CAD build for the part. Positions are in the model's coordinates, mm. A direction names the side the tool comes from. Round coordinates to 2 decimals unless told otherwise and drop trailing zeros. Write each loop counter-clockwise with the first axis right and the second up, starting at its lowest first coordinate (ties: lowest second). Pieces come first, ordered by that corner, then holes. Notation, with made-up numbers: (19, 63) -> (71, 63) arc R31 cw to (71, 92) -> close; hole circle Ø7 at (34, 78). An arc over 180 degrees is marked (long way). Put each result on its own line as item: value. Start each with the question number.
1. 3-axis set-ups, long thin cutter, end or side, ignore diameter. For faces 1 (the flat face through (-7, -1, -1)), 2 (the cylindrical face through (-15.65, -0.06, -1.23)), 3 (the cylindrical face through (-6.604, 2.421, 1.183)), 4 (the cylindrical face through (15.65, 0.06, -1.23)), 5 (the cylindrical face through (-0.73, -3.32, -1.23)): which of +Z, -Z, +X, -X, +Y, -Y reach the whole face in a straight line?
2. Pull direction Y, two halves, no side cores. Call faces 6 (the cylindrical face through (6.604, -2.421, 1.183)), 7 (the cylindrical face through (-3.918, 4.953, -0.873)), 8 (the flat face through (0, 0, -2.5)): pulls with the +Y half, pulls with the -Y half, needs draft (parallel to the pull), parting line crosses it, or undercut.
3. Saw through at B-B on y = -9.5. List the corners of the cut face in (x, z), and give its area (3 significant figures).
4. Drill centre lines: line 1 (Y direction, x = -9.5, z = -0.25); line 2 (X direction, y = 4.5, z = -1.4); line 3 (Z direction, x = 1.5, y = 15.5). Where is each one in solid material? Low to high. Write a range as from..to.
5. Flat gauge pins, fed straight in: P1, Ø2, axis at x = 0.5, z = -0.5, coming from the +Y side; P2, Ø1, axis at y = -6, z = -1, coming from the +X side; P3, Ø2, axis at x = 9, z = -1, coming from the -Y side. Where does each tip first touch, or does it go through?
6. Saw through at A-A on x = -9.5. List the corners of the cut face in (y, z).
7. Saw through at D-D on x = -14.5. List the corners of the cut face in (y, z), and give its area (3 significant figures).
8. Saw through at C-C on x = 0. List the corners of the cut face in (y, z).
from build123d import *

# Parameters (mm, degrees)
F1_DEPTH = 2.5
F2_R     = 2.5
F2_R_2   = 3.5
F3_DEPTH = 1
F4_DEPTH = 25
F6_DEPTH = 2.4
F7_DEPTH = 0.8
F8_ANGLE = 180


with BuildPart() as f1:
    # F0 (on Top) → F1 (new body)
    with BuildSketch(Plane.XY):
        with BuildLine():
            ThreePointArc((-17.7467741935, 3.8045375176), (-15.65, 0), (-17.7467741935, -3.8045375176))
            ThreePointArc((-17.7467741935, -3.8045375176), (0, -18.15), (17.7467741935, -3.8045375176))
            ThreePointArc((17.7467741935, -3.8045375176), (15.65, 0), (17.7467741935, 3.8045375176))
            ThreePointArc((17.7467741935, 3.8045375176), (0, 18.15), (-17.7467741935, 3.8045375176))
        make_face()
        with BuildLine():
            ThreePointArc((2.4959380946, -2.3087427375), (5.3934479575, -2.1979674519), (5.5, -5.0956356923))
            ThreePointArc((5.5, -5.0956356923), (1.7016498657, -7.3374880505), (-2.7, -7.0566959612))
            ThreePointArc((-2.7, -7.0566959612), (-3.9459149151, -4.3705658168), (-1.241297598, -3.1653088749))
            ThreePointArc((-1.241297598, -3.1653088749), (0.7595769091, -3.3140674283), (2.4959380946, -2.3087427375))
        make_face(mode=Mode.SUBTRACT)
        with BuildLine():
            ThreePointArc((-8.7553190403, 9.1305469991), (0.952140072, 12.6141162704), (10.0266934622, 7.7128411247))
            ThreePointArc((10.0266934622, 7.7128411247), (9.5115151335, 3.7722871727), (5.5712685972, 4.2898114644))
            Line((5.5712685972, 4.2898114644), (5.5118136083, 4.3702173366))
            ThreePointArc((5.5118136083, 4.3702173366), (3.8930445069, 4.946510168), (2.7952312611, 3.6246429626))
            ThreePointArc((2.7952312611, 3.6246429626), (2.3794320778, 2.9889401783), (1.6198224227, 2.9893436268))
            ThreePointArc((1.6198224227, 2.9893436268), (-0.1325337371, 3.3974159016), (-1.8477750037, 2.8540720972))
            ThreePointArc((-1.8477750037, 2.8540720972), (-4.009187674, 2.5898113989), (-5.5508583046, 4.1275988078))
            ThreePointArc((-5.5508583046, 4.1275988078), (-5.9755788699, 4.654107591), (-6.6382950389, 4.7897775457))
            ThreePointArc((-6.6382950389, 4.7897775457), (-9.2794977325, 6.1882728138), (-8.7553190403, 9.1305469991))
        make_face(mode=Mode.SUBTRACT)
    extrude(amount=F1_DEPTH)

    # F2 (on face) → F3 (cut)
    with BuildSketch(Plane(origin=(0, 0, 0), x_dir=(1, 0, 0), z_dir=(0, 0, -1))):
        with BuildLine():
            ThreePointArc((9.0125481144, -3.4658895913), (11.7960747375, -2.6415981526), (13, 0))
            ThreePointArc((13, 0), (7.5843636972, 2.9292213224), (8.0969499684, -3.2064701166))
            ThreePointArc((8.0969499684, -3.2064701166), (8.5658137707, -3.297127868), (9.0125481144, -3.4658895913))
        make_face()
        with Locations((9.5, 0)):
            Circle(F2_R, mode=Mode.SUBTRACT)
        with Locations((-9.5, 0)):
            Circle(F2_R_2)
        with Locations((-9.5, 0)):
            Circle(F2_R, mode=Mode.SUBTRACT)
    extrude(amount=-F3_DEPTH, mode=Mode.SUBTRACT)

    # F2 (on face) → F4 (cut)
    with BuildSketch(Plane(origin=(0, 0, 0), x_dir=(1, 0, 0), z_dir=(0, 0, -1))):
        with Locations((9.5, 0)):
            Circle(F2_R)
        with Locations((-9.5, 0)):
            Circle(F2_R)
    extrude(amount=-F4_DEPTH, mode=Mode.SUBTRACT)

    # F5 (on face) → F6 (join)
    with BuildSketch(Plane(origin=(0, 0, 0), x_dir=(1, 0, 0), z_dir=(0, 0, -1))):
        with BuildLine():
            ThreePointArc((6.0601535804, -3.7943429711), (6.2633893685, -3.4485436953), (6.4469143417, -3.0918918919))
            ThreePointArc((6.4469143417, -3.0918918919), (6.6042114466, -2.4108440907), (6.4561602608, -1.7277267266))
            ThreePointArc((6.4561602608, -1.7277267266), (6.4124110495, -1.6482701455), (6.3707355238, -1.5677065536))
            ThreePointArc((6.3707355238, -1.5677065536), (4.9243798524, -0.8019946659), (3.5615820489, -1.7081081081))
            ThreePointArc((3.5615820489, -1.7081081081), (3.1023693948, -2.4449548335), (2.4932688314, -3.0636759839))
            ThreePointArc((2.4932688314, -3.0636759839), (2.7026586012, -3.3127187828), (2.7952312611, -3.6246429626))
            ThreePointArc((2.7952312611, -3.6246429626), (3.8930445069, -4.946510168), (5.5118136083, -4.3702173366))
            Line((5.5118136083, -4.3702173366), (5.5712685972, -4.2898114644))
            ThreePointArc((5.5712685972, -4.2898114644), (5.8003063385, -4.0268771571), (6.0601535804, -3.7943429711))
        make_face()
        with BuildLine():
            ThreePointArc((3.8959765845, -5.9953203795), (5.0982553244, -5.0130123326), (6.0601535804, -3.7943429711))
            ThreePointArc((6.0601535804, -3.7943429711), (5.8003063385, -4.0268771571), (5.5712685972, -4.2898114644))
            Line((5.5712685972, -4.2898114644), (5.5118136083, -4.3702173366))
            ThreePointArc((5.5118136083, -4.3702173366), (3.8930445069, -4.946510168), (2.7952312611, -3.6246429626))
            ThreePointArc((2.7952312611, -3.6246429626), (2.7026586012, -3.3127187828), (2.4932688314, -3.0636759839))
            ThreePointArc((2.4932688314, -3.0636759839), (2.3261145429, -3.192442816), (2.1523227285, -3.3121000698))
            ThreePointArc((2.1523227285, -3.3121000698), (1.6825395016, -5.5255371527), (3.8959765845, -5.9953203795))
        make_face()
        with BuildLine():
            ThreePointArc((-3.8662701246, 6.0141635011), (-3.8811751433, 6.0048235859), (-3.8959765845, 5.9953203795))
            ThreePointArc((-3.8959765845, 5.9953203795), (-5.3713427021, 4.7192348508), (-6.4469143417, 3.0918918919))
            ThreePointArc((-6.4469143417, 3.0918918919), (-6.6042114466, 2.4108440907), (-6.4561602608, 1.7277267266))
            ThreePointArc((-6.4561602608, 1.7277267266), (-6.4124110495, 1.6482701455), (-6.3707355238, 1.5677065536))
            ThreePointArc((-6.3707355238, 1.5677065536), (-4.9243798524, 0.8019946659), (-3.5615820489, 1.7081081081))
            ThreePointArc((-3.5615820489, 1.7081081081), (-3.0956887113, 2.4534081198), (-2.4765181166, 3.0772322009))
            ThreePointArc((-2.4765181166, 3.0772322009), (-3.8784449822, 4.2111223181), (-3.8662701246, 6.0141635011))
        make_face()
        with BuildLine():
            ThreePointArc((-2.1523227285, 3.3121000698), (-1.6730362952, 5.5107357114), (-3.8662701246, 6.0141635011))
            ThreePointArc((-3.8662701246, 6.0141635011), (-3.8784449822, 4.2111223181), (-2.4765181166, 3.0772322009))
            ThreePointArc((-2.4765181166, 3.0772322009), (-2.3173978125, 3.1987759188), (-2.1523227285, 3.3121000698))
        make_face()
    extrude(amount=F6_DEPTH)

    # F7 (cut): faces of the model
    f7_faces = [f1.faces().sort_by_distance(p)[0] for p in [
        (2.880203055, 4.9455389585, 0),
        (-2.7641546482, -4.7635377555, 0),
    ]]
    extrude(f7_faces, amount=-F7_DEPTH, mode=Mode.SUBTRACT)


with BuildPart() as f1_1:
    # F8: moved
    add(f1.part.rotate(Axis((0, 0, 0), (0, -1, 0)), F8_ANGLE))


solid = f1_1.part
Return value:
1. face 1: +Z
1. face 2: +Z, -Z, -X
1. face 3: +Z, -X
1. face 4: +Z, -Z, +X
1. face 5: +Z, -Z
2. face 6: parting line crosses it
2. face 7: undercut
2. face 8: needs draft
3. outline: (-15.47, -2.5) -> (15.47, -2.5) -> (15.47, 0) -> (-15.47, 0) -> close
3. area: 77.3 mm^2
4. line 1: y = -15.47..-3.5, 3.5..3.76, 8.35..15.47
4. line 2: x = -17.58..-10.18, -5.41..-3.17, 5.78..17.58
4. line 3: z = -2.5..0
5. P1: stops at y = 18.15
5. P2: stops at x = 17.3
5. P3: stops at y = -16.29
6. outline: (-15.47, -2.5) -> (-2.5, -2.5) -> (-2.5, -1) -> (-3.5, -1) -> (-3.5, 0) -> (-15.47, 0) -> close; (2.5, -2.5) -> (3.76, -2.5) -> (3.76, 0) -> (3.5, 0) -> (3.5, -1) -> (2.5, -1) -> close; (8.35, -2.5) -> (15.47, -2.5) -> (15.47, 0) -> (8.35, 0) -> close
7. outline: (-10.92, -2.5) -> (10.92, -2.5) -> (10.92, 0) -> (-10.92, 0) -> close
7. area: 54.6 mm^2
8. outline: (-18.15, -2.5) -> (-7.54, -2.5) -> (-7.54, 0) -> (-18.15, 0) -> close; (-3.4, -2.5) -> (3.4, -2.5) -> (3.4, 0) -> (-3.4, 0) -> close; (12.65, -2.5) -> (18.15, -2.5) -> (18.15, 0) -> (12.65, 0) -> close
